```python
from build123d import *

# Parameters (mm, degrees)
SKETCH1_R           = 25.4
EXTRUDE1_DEPTH      = 22.225
EXTRUDE1_DEPTH_BACK = 88.9
CUT_EXTRUDE1_REACH  = 90.9
SKETCH2_R           = 25.4
SKETCH2_R_2         = 23.622
CUT_EXTRUDE3_REACH  = 31.464
CUT_EXTRUDE3_START  = -7.239
CUT_EXTRUDE4_DEPTH  = 7.239
SKETCH20_R          = 8.6614
CUT_EXTRUDE5_DEPTH  = 0.254
CHAMFER1_SIZE       = 0.762
EXTRUDE3_DEPTH      = 7.112
CIRPATTERN1_COUNT   = 4


with BuildPart() as part:
    # Sketch1 → Extrude1 (new body, two sides)
    with BuildSketch(Plane(origin=(0, 0, 0), x_dir=(0, 0, -1), z_dir=(1, 0, 0))) as extrude1_sk:
        Circle(SKETCH1_R)
    extrude(amount=EXTRUDE1_DEPTH)
    extrude(extrude1_sk.sketch, amount=-EXTRUDE1_DEPTH_BACK)

    # Sketch2 → Cut-Extrude1 (cut, up to next)
    with BuildSketch(Plane(origin=(0, 0, 0), x_dir=(0, 0, -1), z_dir=(1, 0, 0)), mode=Mode.PRIVATE) as cut_extrude1_sk1:
        Circle(SKETCH2_R)
        Circle(SKETCH2_R_2, mode=Mode.SUBTRACT)
    cut_extrude1_tool1 = extrude(cut_extrude1_sk1.sketch, amount=-CUT_EXTRUDE1_REACH, mode=Mode.PRIVATE) & part.part
    add(cut_extrude1_tool1.solids().sort_by_distance((0, 0, 24.68158))[0], mode=Mode.SUBTRACT)

    # Sketch4 → Cut-Extrude3 (cut, up to next)
    with BuildSketch(Plane.ZY.offset(CUT_EXTRUDE3_START), mode=Mode.PRIVATE) as cut_extrude3_sk1:
        with BuildLine():
            Line((20.5105, -14.982636275), (20.5105, 14.982636275))
            ThreePointArc((20.5105, 14.982636275), (25.4, 0), (20.5105, -14.982636275))
        make_face()
    cut_extrude3_tool1 = extrude(cut_extrude3_sk1.sketch, amount=-CUT_EXTRUDE3_REACH, mode=Mode.PRIVATE) & part.part
    add(cut_extrude3_tool1.solids().sort_by_distance((7.239, 0, 22.48339))[0], mode=Mode.SUBTRACT)
    # Sketch4 → Cut-Extrude3 (cut, up to next)
    with BuildSketch(Plane.ZY.offset(CUT_EXTRUDE3_START), mode=Mode.PRIVATE) as cut_extrude3_sk2:
        with BuildLine():
            Line((7.774889797, 24.1808), (-7.774889797, 24.1808))
            ThreePointArc((-7.774889797, 24.1808), (0, 25.4), (7.774889797, 24.1808))
        make_face()
    cut_extrude3_tool2 = extrude(cut_extrude3_sk2.sketch, amount=-CUT_EXTRUDE3_REACH, mode=Mode.PRIVATE) & part.part
    add(cut_extrude3_tool2.solids().sort_by_distance((7.239, 24.669497, 0))[0], mode=Mode.SUBTRACT)
    # Sketch4 → Cut-Extrude3 (cut, up to next)
    with BuildSketch(Plane.ZY.offset(CUT_EXTRUDE3_START), mode=Mode.PRIVATE) as cut_extrude3_sk3:
        with BuildLine():
            Line((-20.5105, -14.982636275), (-20.5105, 14.982636275))
            ThreePointArc((-20.5105, 14.982636275), (-25.4, 0), (-20.5105, -14.982636275))
        make_face()
    cut_extrude3_tool3 = extrude(cut_extrude3_sk3.sketch, amount=-CUT_EXTRUDE3_REACH, mode=Mode.PRIVATE) & part.part
    add(cut_extrude3_tool3.solids().sort_by_distance((7.239, 0, -22.48339))[0], mode=Mode.SUBTRACT)

    # Sketch19 → Cut-Extrude4 (cut)
    with BuildSketch(Plane(origin=(7.239, 0, 0), x_dir=(0, 0, -1), z_dir=(1, 0, 0))):
        with BuildLine():
            Line((-7.774889797, 24.1808), (7.774889797, 24.1808))
            ThreePointArc((7.774889797, 24.1808), (0, 25.4), (-7.774889797, 24.1808))
        make_face()
    extrude(amount=-CUT_EXTRUDE4_DEPTH, mode=Mode.SUBTRACT)

    # Sketch6 → Cut-Revolve2 (revolve, cut)
    with BuildSketch(Plane.XY, mode=Mode.PRIVATE) as cut_revolve2_sk:
        Polygon((2.061041849, 50.8), (22.225, 15.875), (22.225, 50.8), align=None)
    revolve(cut_revolve2_sk.sketch.rotate(Axis((1.052843941, 0, 0), (1, 0, 0)), 270), axis=Axis((1.052843941, 0, 0), (1, 0, 0)), mode=Mode.SUBTRACT)  # turned: the seam where the file's is

    # S2D0002 → Cut-Revolve3 (revolve, cut)
    with BuildSketch(Plane(origin=(5.969, 23.9268, 0), x_dir=(1, 0, 0), z_dir=(0, 0, 1)), mode=Mode.PRIVATE) as cut_revolve3_sk:
        Polygon((0, 0), (4.5466, 0), (4.106586662, -2.0701), (3.4544, -2.722286662), (3.4544, -12.192), (0, -12.192), align=None)
    revolve(cut_revolve3_sk.sketch.rotate(Axis((5.969, 11.1252, 0), (0, 1, 0)), 90), axis=Axis((5.969, 11.1252, 0), (0, 1, 0)), mode=Mode.SUBTRACT)  # turned: the seam where the file's is

    # Sketch20 → Cut-Extrude5 (cut)
    with BuildSketch(Plane(origin=(0, 24.1808, 0), x_dir=(1, 0, 0), z_dir=(0, 1, 0))):
        with Locations((5.969, 0)):
            Circle(SKETCH20_R)
    extrude(amount=-CUT_EXTRUDE5_DEPTH, mode=Mode.SUBTRACT)

    # Sketch9 → Cut-Revolve5 (revolve, cut)
    with BuildSketch(Plane.XY, mode=Mode.PRIVATE) as cut_revolve5_sk:
        Polygon((0, 23.622), (0, 22.606), (-3.302, 22.606), (-4.318, 23.622), align=None)
    revolve(cut_revolve5_sk.sketch.rotate(Axis((-4.5339, 0, 0), (1, 0, 0)), 90), axis=Axis((-4.5339, 0, 0), (1, 0, 0)), mode=Mode.SUBTRACT)  # turned: the seam where the file's is

    # Sketch11 → Cut-Revolve7 (revolve, cut)
    with BuildSketch(Plane.XY, mode=Mode.PRIVATE) as cut_revolve7_sk:
        Polygon((-88.9, 23.622), (-88.9, 22.606), (-86.36, 22.606), (-85.344, 23.622), align=None)
    revolve(cut_revolve7_sk.sketch.rotate(Axis((-89.0778, 0, 0), (1, 0, 0)), 90), axis=Axis((-89.0778, 0, 0), (1, 0, 0)), mode=Mode.SUBTRACT)  # turned: the seam where the file's is

    # Chamfer1
    chamfer1_edges = [part.edges().sort_by_distance(p)[0] for p in [
        (-88.9, 0, -22.606),
    ]]
    chamfer(chamfer1_edges, length=CHAMFER1_SIZE)

    # Sketch12 → Revolve1 (revolve)
    with BuildSketch(Plane(origin=(0, 0, 0), x_dir=(0, -1, 0), z_dir=(0, 0, 1)), mode=Mode.PRIVATE) as revolve1_sk:
        with BuildLine():
            Line((0, 22.225), (0, 60.0964))
            Line((0, 60.0964), (10.0965, 60.0964))
            ThreePointArc((10.0965, 60.0964), (10.81492049, 59.79882049), (11.1125, 59.0804))
            Line((11.1125, 59.0804), (11.1125, 22.225))
            Line((11.1125, 22.225), (0, 22.225))
        make_face()
    revolve(revolve1_sk.sketch.rotate(Axis((20.33143, 0, 0), (1, 0, 0)), 270), axis=Axis((20.33143, 0, 0), (1, 0, 0)))  # turned: the seam where the file's is

    # S2D0001 → Cut-Revolve8 (revolve, cut)
    with BuildSketch(Plane(origin=(60.0964, -5.7531, 0), x_dir=(0, -1, 0), z_dir=(0, 0, 1)), mode=Mode.PRIVATE) as cut_revolve8_sk:
        Polygon((0, 0), (0, -17.018), (-5.7531, -20.474811227), (-5.7531, 0), align=None)
    revolve(cut_revolve8_sk.sketch.rotate(Axis((38.597848211, 0, 0), (1, 0, 0)), 270), axis=Axis((38.597848211, 0, 0), (1, 0, 0)), mode=Mode.SUBTRACT)  # turned: the seam where the file's is

    # S2D0003 → Extrude3 (add)
    with BuildSketch(Plane.ZX.offset(23.9268)):
        Polygon((-4.12811216, 13.1191), (4.12811216, 13.1191), (8.256224319, 5.969), (4.12811216, -1.1811), (-4.12811216, -1.1811), (-8.256224319, 5.969), align=None)
    extrude(amount=EXTRUDE3_DEPTH)

    # Sketch16 → Revolve2 (revolve)
    with BuildSketch(Plane(origin=(0, 0, 0), x_dir=(0, -1, 0), z_dir=(0, 0, 1)), mode=Mode.PRIVATE) as revolve2_sk:
        Polygon((-31.0388, 11.049), (-32.5628, 11.049), (-33.0327, 11.5189), (-40.9575, 11.5189), (-41.4274, 11.049), (-42.9514, 11.049), (-45.0088, 9.498637897), (-45.0088, 7.5565), (-31.0388, 7.5565), align=None)
    revolve(revolve2_sk.sketch.rotate(Axis((5.969, 45.7073, 0), (0, -1, 0)), 90), axis=Axis((5.969, 45.7073, 0), (0, -1, 0)))  # turned: the seam where the file's is

    # Sketch17 → Cut-Revolve9 (revolve, cut)
    with BuildSketch(Plane(origin=(56.134, 7.857724106, -7.857724106), x_dir=(-1, 0, 0), z_dir=(0, -0.707106781, -0.707106781)), mode=Mode.PRIVATE) as cut_revolve9_sk:
        Polygon((0, 0), (2.413, 0), (0, -2.413), align=None)
    cut_revolve9 = revolve(cut_revolve9_sk.sketch.rotate(Axis((56.134, 6.06616301, -6.06616301), (0, 0.707106781, -0.707106781)), 90), axis=Axis((56.134, 6.06616301, -6.06616301), (0, 0.707106781, -0.707106781)), mode=Mode.SUBTRACT)  # turned: the seam where the file's is

    # CirPattern1: Cut-Revolve9 ×4 about axis
    cirpattern1_axis = Axis((-88.901, 0, 0), (1, 0, 0))
    for i in range(1, CIRPATTERN1_COUNT):
        add(cut_revolve9.rotate(cirpattern1_axis, i * 360 / CIRPATTERN1_COUNT), mode=Mode.SUBTRACT)


solid = part.part
```
Check sheet for the modelled part. Datum: model origin and axes. Units: mm. A direction names the side the tool comes from. Coordinates: 2 decimals unless noted, no trailing zeros. Loops run counter-clockwise (first coordinate to the right, second up) from the corner with the lowest first, then second, coordinate; pieces in that order, holes last.
1) Access from +Z, -Z, +X, -X, +Y, -Y to the whole of each face (thin tool, end or side, straight path). Record for faces 1 (the face through (13, 0, 20.51)), 2 (the face through (7.52, 37.93, -0.34)), 3 (the face through (-87.24, 22.07, -4.9)).
2) Sectioned sample at A-A (y = 28). Record the boundary of the cut face in (x, z), and give its area (3 significant figures).
3) Sectioned sample at C-C (x = -43). Record the boundary of the cut face in (y, z), and give its area (3 significant figures).
4) Material ranges on probe 1 along X at (y, z) = (15.5, 0) (3 decimals); probe 2 along X at (y, z) = (34.25, 0); probe 3 along Y at (x, z) = (55, 0), recorded low to high.
5) Release check for a two-part mould opening along Z. For faces 4 (the face through (40.174, -0.276, 0.876)), 5 (the face through (0.932, 42.2, -0.661)), 6 (the face through (13, 0, -20.51)), 7 (the face through (6, 31.039, 0)) record: released by +Z, released by -Z, zero draft, split by the parting line, or undercut.
6) Gauge pin test, flat ends, axial feed: pin 1 (10 mm diameter, centred on x = -12, z = -11, fed in from +Y); pin 2 (10 mm diameter, centred on x = 5, z = 2, fed in from -Y); pin 3 (8 mm diameter, centred on y = 28, z = -1, fed in from +X). Record the tip position at first contact, or that the pin passes through.
7) Sectioned sample at B-B (y = 37). Record the boundary of the cut face in (x, z) (1 decimal), and give its area (3 significant figures).
Check sheet entries:
1. face 1: +Z, +X, +Y, -Y
1. face 2: +Y
1. face 3: -X
2. outline: (-1.18, -4.13) - (5.97, -8.26) - (13.12, -4.13) - (13.12, 4.13) - (5.97, 8.26) - (-1.18, 4.13) - close
2. area: 177 mm2
3. outline: circle Ø47.24 at (0, 0)
3. area: 1,750 mm2
4. probe 1: x = -88.9 to 2.515, 9.423 to 22.225
4. probe 2: x = 0.42 to 4.38, 7.56 to 11.52
4. probe 3: y = -11.11 to -5.75, 5.75 to 11.11
5. face 4: undercut
5. face 5: split by the parting line
5. face 6: released by -Z
5. face 7: undercut
6. pin 1: stops at y = 22.85
6. pin 2: stops at y = -25.4
6. pin 3: stops at x = 17.52
7. outline: circle Ø11.1 at (6, 0); hole circle Ø3.2 at (6, 0)
7. area: 88.8 mm2
